Part model, mm, in its own coordinate system. Coordinates: 2 decimals unless noted, no trailing zeros. Loops run counter-clockwise (first coordinate to the right, second up) from the corner with the lowest first, then second, coordinate; pieces in that order, holes last. Notation, with made-up numbers: (81, 80.25) - (103, 80.25) arc R11 ccw to (103, 87.25) - close; hole circle Ø5 at (-11, 4). An arc over 180 degrees is marked (long way). Use a Markdown table: item, result. Add a question column.
1) Probe probe 1 along X at (y, z) = (2, 0); probe 2 along Z at (x, y) = (-28.5, 5.5); probe 3 along Z at (x, y) = (-28, 4). List the from-to ranges inside material, lowest first. Write a range as [from, to].
2) Band-saw the part on A-A (y = 4). Give the cut face in (x, z), plus the area to 3 significant figures.
3) Band-saw the part on C-C (z = -22). Give the cut face in (x, y).
4) Band-saw the part on B-B (x = -36). Give the cut face in (y, z), plus the area to 3 significant figures.
5) Band-saw the part on D-D (x = -7). Give the cut face in (y, z).
6) Drop flat-ended pins along their axis: P1, Ø1.9, axis at y = 4, z = 11.5, coming from the +X side; P2, Ø3, axis at y = 3, z = 10, coming from the -X side; P3, Ø1.9, axis at y = 4, z = -20, coming from the -X side. Give the stop position or say it passes through.
from build123d import *

# Parameters (mm, degrees)
SKETCH1_R           = 63.5
SKETCH1_W           = 17.78
SKETCH1_H           = 6.35
SKETCH1_W_2         = 6.35
SKETCH1_R_2         = 1.27
BOSS_EXTRUDE3_DEPTH = 6.35


with BuildPart() as part:
    # Sketch1 → Boss-Extrude3 (new body)
    with BuildSketch(Plane(origin=(0, 0, 0), x_dir=(1, 0, 0), z_dir=(0, 1, 0))):
        with Locations(Location((0, 0, 0), (0, 0, 270))):
            Circle(SKETCH1_R)
        Polygon((-34.262799333, -7.326577006), (-27.912799333, -7.326577006), (-27.912799333, -13.676577006), (-34.262799333, -13.676577006), (-40.612799333, -13.676577006), (-40.612799333, -7.326577006), align=None, mode=Mode.SUBTRACT)
        with Locations((21.870627403, -34.682199949)):
            Rectangle(SKETCH1_W, SKETCH1_H, mode=Mode.SUBTRACT)
        with Locations((20.20048917, -10.501577006)):
            Rectangle(SKETCH1_W_2, SKETCH1_H, mode=Mode.SUBTRACT)
        Polygon((-27.912799333, 5.373422994), (-34.262799333, 5.373422994), (-40.612799333, 5.373422994), (-40.612799333, 11.723422994), (-34.262799333, 11.723422994), (-27.912799333, 11.723422994), align=None, mode=Mode.SUBTRACT)
        with Locations((-4.076334422, 20.437374514)):
            Rectangle(SKETCH1_W, SKETCH1_H, mode=Mode.SUBTRACT)
        with Locations(Location((0, 0, 0), (0, 0, 270))):
            Circle(SKETCH1_R_2, mode=Mode.SUBTRACT)
        with Locations((20.20048917, 8.548422994)):
            Rectangle(SKETCH1_W_2, SKETCH1_H, mode=Mode.SUBTRACT)
    extrude(amount=BOSS_EXTRUDE3_DEPTH)


solid = part.part
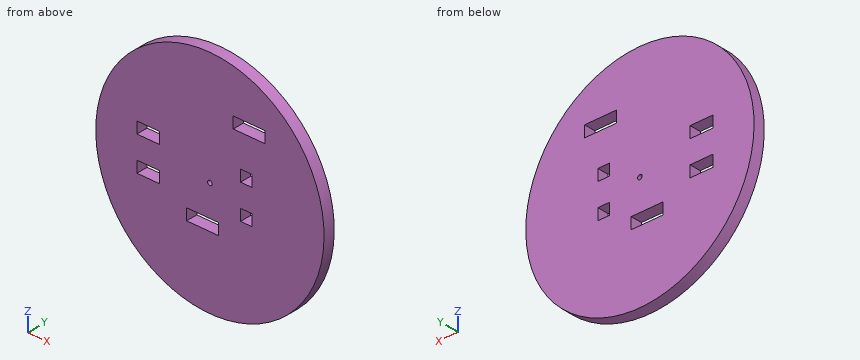
Answer block:
| question | item | result |
|---|---|---|
| 1 | probe 1 | [-63.5, -1.27], [1.27, 63.5] |
| 1 | probe 2 | [-56.75, -11.72], [-5.37, 7.33], [13.68, 56.75] |
| 1 | probe 3 | [-56.99, -11.72], [-5.37, 7.33], [13.68, 56.99] |
| 2 | outline | circle Ø127 at (0, 0); hole (-40.61, -11.72) - (-27.91, -11.72) - (-27.91, -5.37) - (-40.61, -5.37) - close; hole (-40.61, 7.33) - (-27.91, 7.33) - (-27.91, 13.68) - (-40.61, 13.68) - close; hole (-12.97, -23.61) - (4.81, -23.61) - (4.81, -17.26) - (-12.97, -17.26) - close; hole circle Ø2.54 at (0, 0); hole (12.98, 31.51) - (30.76, 31.51) - (30.76, 37.86) - (12.98, 37.86) - close; hole (17.03, -11.72) - (23.38, -11.72) - (23.38, -5.37) - (17.03, -5.37) - close; hole (17.03, 7.33) - (23.38, 7.33) - (23.38, 13.68) - (17.03, 13.68) - close |
| 2 | area | 12,200 mm2 |
| 3 | outline | (-59.57, 0) - (-12.97, 0) - (-12.97, 6.35) - (-59.57, 6.35) - close; (4.81, 0) - (59.57, 0) - (59.57, 6.35) - (4.81, 6.35) - close |
| 4 | outline | (0, -52.31) - (6.35, -52.31) - (6.35, -11.72) - (0, -11.72) - close; (0, -5.37) - (6.35, -5.37) - (6.35, 7.33) - (0, 7.33) - close; (0, 13.68) - (6.35, 13.68) - (6.35, 52.31) - (0, 52.31) - close |
| 4 | area | 584 mm2 |
| 5 | outline | (0, -63.11) - (6.35, -63.11) - (6.35, -23.61) - (0, -23.61) - close; (0, -17.26) - (6.35, -17.26) - (6.35, 63.11) - (0, 63.11) - close |
| 6 | P1 | x = 62.62 |
| 6 | P2 | x = -62.93 |
| 6 | P3 | x = -60.58 |
